Build history of the part. All positions in model axes, mm. A direction names the side the tool comes from. Give positions to 0.01 mm unless a question says otherwise; leave off trailing zeros. Order: outer loops, then holes, each group sorted by start corner. A loop starts at its lowest first (then second) coordinate and runs counter-clockwise, first axis right, second up. Notation, with made-up numbers: M 74,-2.5 L 131,-2.5 A16 cw 131,10.5 Z; hole C 27,72.5 d11. An arc over 180 degrees is marked long. Use CSV: the item, a comma, the result in double quotes. Start each with the question number.
Item 1: Pin check, flat tips, straight feed: P1, Ø0.7, axis at y = -174.5, z = -99, coming from the -X side; P2, Ø0.7, axis at y = 174.5, z = -99.5, coming from the +X side; P3, Ø1.1, axis at y = 174.5, z = -99.5, coming from the -X side. Stop position of each tip, or through.
Item 2: Two-plate mould, pull along X, no slides. Class faces 1 (the flat face through (188.756, 2.439, -60.178)), 2 (the flat face through (198.75, 91.68, -51.61)), 3 (the flat face through (-189.59, 2.45, -61.6)): pulls with the +X half, pulls with the -X half, needs draft (parallel to the pull), parting line crosses it, or undercut.
Item 3: Which spindle directions (+Z, -Z, +X, -X, +Y, -Y) get a long thin tool onto all of the face, cutting with end or side? Do faces 4 (the flat face through (-188.756, 2.439, -60.178)), 5 (the flat face through (189.59, 2.45, -61.6)). Say none if no direction does.
Item 4: Band-saw the part on A-A on z = -93. Write the cut outline in (x, y).
Item 5: Band-saw the part on D-D on z = -28. Write the cut outline in (x, y), plus the area to 3 significant figures.
Item 6: Wall check: line 1 along Z through (x, y) = (-86.5, -134); line 2 along X through (y, z) = (-26, -55); line 3 along X through (y, z) = (22, -92). Give the ranges that are in metal, low to high.
Item 7: Band-saw the part on B-B on y = 66.5. Write the cut outline in (x, z), plus the area to 3 significant figures.
Item 8: Band-saw the part on C-C on x = -44.5. Write the cut outline in (y, z), plus the area to 3 significant figures.
from build123d import *

# Parameters (mm, degrees)
SKETCH003_W  = 300
SKETCH003_H  = 350
PAD003_DEPTH = 1.6
PAD004_DEPTH = 1.6
SKETCH005_R  = 4
POCKET_DEPTH = 348.954325


with BuildPart() as part:
    # Sketch003 → Pad003 (new body)
    with BuildSketch(Plane.XY):
        Rectangle(SKETCH003_W, SKETCH003_H)
    extrude(amount=PAD003_DEPTH)

    with BuildSketch(Plane(origin=(-150, 0, 0), x_dir=(0.717792, 0, -0.696258), z_dir=(0.696258, 0, 0.717792))):
        Polygon((0, -175), (0, 175), (-139.316187, 6), (-139.316187, -6), align=None)
    pad004 = extrude(amount=PAD004_DEPTH)

    # Mirrored001: Pad004 across YZ
    add(pad004.mirror(Plane.YZ))

    with BuildSketch(Plane(origin=(-150, 0, 0), x_dir=(0.717792, 0, -0.696258), z_dir=(0.696258, 0, 0.717792))):
        with Locations((-32, 9.5)):
            Circle(SKETCH005_R)
        with Locations((-32, -9.5)):
            Circle(SKETCH005_R)
    extrude(amount=POCKET_DEPTH, mode=Mode.SUBTRACT)


with BuildPart() as part_1:
    # Body002 placement: moved
    add(part.part.moved(Location((0, 0, -100))))


solid = part_1.part
Model answer:
1,P1,"stops at x = -150.13"
1,P2,"stops at x = 150.5"
1,P3,"stops at x = -150.62"
2,face 1,"undercut"
2,face 2,"pulls with the +X half"
2,face 3,"pulls with the -X half"
3,face 4,"+Z, +Y, -Y"
3,face 5,"-Z, +X, +Y, -Y"
4,outline,"M -157.22,-162.8 L -154.92,-164.81 L -154.92,164.81 L -157.22,162.8 Z; M 154.92,-164.81 L 157.22,-162.8 L 157.22,162.8 L 154.92,164.81 Z"
5,outline,"M -224.23,-49.56 L -221.93,-51.56 L -221.93,51.56 L -224.23,49.56 Z; M 221.93,-51.56 L 224.23,-49.56 L 224.23,49.56 L 221.93,51.56 Z"
5,area,"465 mm^2"
6,line 1,"z = -100 to -98.4"
6,line 2,"x = -196.39 to -194.09, 194.09 to 196.39"
6,line 3,"x = -158.25 to -155.95, 155.95 to 158.25"
7,outline,"M -214.2,-37.72 L -150,-100 L 150,-100 L 214.2,-37.72 L 213.09,-36.58 L 149.35,-98.4 L -149.35,-98.4 L -213.09,-36.58 Z"
7,area,"764 mm^2"
8,outline,"M -175,-100 L 175,-100 L 175,-98.4 L -175,-98.4 Z"
8,area,"560 mm^2"
